Verification items for the finished model (mm, model axes). Give positions to 0.01 mm unless a question says otherwise; leave off trailing zeros. Loops run counter-clockwise (first coordinate to the right, second up) from the corner with the lowest first, then second, coordinate; pieces in that order, holes last. Notation, with made-up numbers: M 50.25,75.5 L 59.25,75.5 A10 ccw 59.25,81.5 Z; hole C 16.25,0.5 d11. An arc over 180 degrees is marked long. Answer in a Markdown table with one row per item.
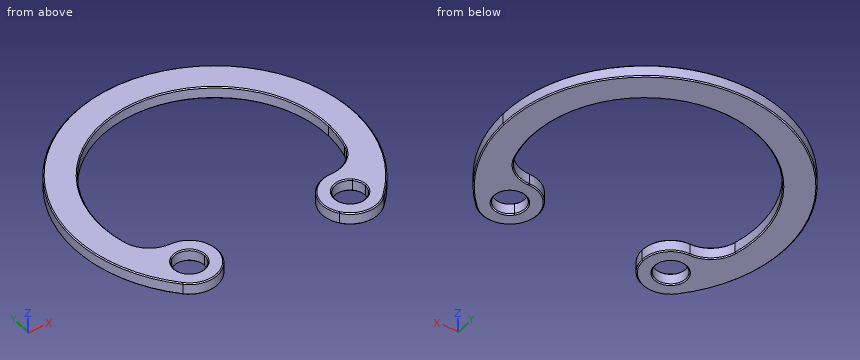
```python
from build123d import *

# Parameters (mm, degrees)
F1_DEPTH = 1.2
F2_R     = 3
F3_SIZE  = 0.1


with BuildPart() as f1:
    # F0 (on Top) → F1 (new body)
    with BuildSketch(Plane.XY):
        with BuildLine():
            ThreePointArc((9.8641395976, -9.8641395976), (12.8881194785, -5.3384338815), (13.95, 0))
            ThreePointArc((13.95, 0), (-5.3384338815, 12.8881194785), (-9.8641395976, -9.8641395976))
            ThreePointArc((-9.8641395976, -9.8641395976), (-10.6786952908, -7.7081070294), (-9.5998734147, -5.6714134412))
            ThreePointArc((-9.5998734147, -5.6714134412), (-2.939720346, 10.7554890306), (11.15, 0))
            ThreePointArc((11.15, 0), (10.7554890306, -2.939720346), (9.5998734147, -5.6714134412))
            ThreePointArc((9.5998734147, -5.6714134412), (10.3985766909, -6.6521228911), (10.6842406102, -7.8842406102))
            ThreePointArc((10.6842406102, -7.8842406102), (10.4711033013, -8.9557542209), (9.8641395976, -9.8641395976))
        make_face()
        with BuildLine():
            ThreePointArc((-5.0842406102, -7.8842406102), (-6.6521228911, -5.3699045296), (-9.5998734147, -5.6714134412))
            ThreePointArc((-9.5998734147, -5.6714134412), (-9.251381225, -6.2237003004), (-8.8711537165, -6.7546377948))
            ThreePointArc((-8.8711537165, -6.7546377948), (-7.2639058858, -6.5185229126), (-6.3842406102, -7.8842406102))
            ThreePointArc((-6.3842406102, -7.8842406102), (-6.4798894748, -8.4113059652), (-6.7546377948, -8.8711537165))
            ThreePointArc((-6.7546377948, -8.8711537165), (-6.2237003004, -9.251381225), (-5.6714134412, -9.5998734147))
            ThreePointArc((-5.6714134412, -9.5998734147), (-5.2350977231, -8.7909059086), (-5.0842406102, -7.8842406102))
        make_face()
        with BuildLine():
            ThreePointArc((-9.5998734147, -5.6714134412), (-10.6786952908, -7.7081070294), (-9.8641395976, -9.8641395976))
            ThreePointArc((-9.8641395976, -9.8641395976), (-7.7081070294, -10.6786952908), (-5.6714134412, -9.5998734147))
            ThreePointArc((-5.6714134412, -9.5998734147), (-6.2237003004, -9.251381225), (-6.7546377948, -8.8711537165))
            ThreePointArc((-6.7546377948, -8.8711537165), (-8.944900782, -8.944900782), (-8.8711537165, -6.7546377948))
            ThreePointArc((-8.8711537165, -6.7546377948), (-9.251381225, -6.2237003004), (-9.5998734147, -5.6714134412))
        make_face()
        with BuildLine():
            ThreePointArc((9.5998734147, -5.6714134412), (5.9043416229, -5.9043416229), (5.6714134412, -9.5998734147))
            ThreePointArc((5.6714134412, -9.5998734147), (6.2237003004, -9.251381225), (6.7546377948, -8.8711537165))
            ThreePointArc((6.7546377948, -8.8711537165), (6.8235804385, -6.8235804385), (8.8711537165, -6.7546377948))
            ThreePointArc((8.8711537165, -6.7546377948), (9.251381225, -6.2237003004), (9.5998734147, -5.6714134412))
        make_face()
        with BuildLine():
            ThreePointArc((5.6714134412, -9.5998734147), (7.7081070294, -10.6786952908), (9.8641395976, -9.8641395976))
            ThreePointArc((9.8641395976, -9.8641395976), (10.4711033013, -8.9557542209), (10.6842406102, -7.8842406102))
            ThreePointArc((10.6842406102, -7.8842406102), (10.3985766909, -6.6521228911), (9.5998734147, -5.6714134412))
            ThreePointArc((9.5998734147, -5.6714134412), (9.251381225, -6.2237003004), (8.8711537165, -6.7546377948))
            ThreePointArc((8.8711537165, -6.7546377948), (9.2499583079, -7.2639058858), (9.3842406102, -7.8842406102))
            ThreePointArc((9.3842406102, -7.8842406102), (8.4113059652, -9.2885917457), (6.7546377948, -8.8711537165))
            ThreePointArc((6.7546377948, -8.8711537165), (6.2237003004, -9.251381225), (5.6714134412, -9.5998734147))
        make_face()
    extrude(amount=F1_DEPTH)

    # F2
    f2_edges = [f1.edges().sort_by_distance(p)[0] for p in [
        (-9.599873, -5.671413, 0.6),
        (9.599873, -5.671413, 0.6),
    ]]
    fillet(f2_edges, radius=F2_R)

    # F3
    f3_edges = [f1.edges().sort_by_distance(p)[0] for p in [
        (-5.297863, -8.956926, 1.2),
        (-9.710143, -4.460557, 1.2),
        (0, 13.95, 1.2),
        (0, 11.15, 1.2),
        (5.297863, -8.956926, 1.2),
        (9.710143, -4.460557, 1.2),
        (-6.897328, -9.013843, 1.2),
        (9.013843, -6.897328, 1.2),
        (0, 11.15, 0),
        (-6.897328, -9.013843, 0),
        (9.013843, -6.897328, 0),
    ]]
    chamfer(f3_edges, length=F3_SIZE)


solid = f1.part
```
Item 1: Scan lines: L1, parallel to Y at x = -8, z = 0.65; L2, parallel to Y at x = 0, z = 0.95; L3, parallel to Y at x = 7, z = 0.95. Record each from-to range of solid material in increasing order. Write a range as [from, to].
Reported:
| item | result |
|---|---|
| L1 | y = [-10.68, -9.38], [-6.39, -5.08], [7.77, 11.43] |
| L2 | y = [11.15, 13.95] |
| L3 | y = [-10.54, -9.1], [-6.67, -5.23], [8.68, 12.07] |
Item 2: Go/stop test with a flat-tipped pin: pin 1 (6 mm diameter, centred on x = -6.5, y = 11.5, fed in from -Z). Record where the tip stops, or that it passes through.
Reported:
| item | result |
|---|---|
| pin 1 | stops at z = 0 |
Item 3: Sectioned sample at B-B (z = 0.65). State how many separate pieces and enclosed holes the cut face has, and give its area (3 significant figures).
Reported:
| item | result |
|---|---|
| separate pieces | 1 |
| enclosed holes | 2 |
| area | 190 mm^2 |
Item 4: Sectioned sample at A-A (x = 0). Record the cut outline in (y, z), and give its area (3 significant figures).
Reported:
| item | result |
|---|---|
| outline | M 11.15,0.1 L 11.25,0 L 13.85,0 L 13.95,0.1 L 13.95,1.1 L 13.85,1.2 L 11.25,1.2 L 11.15,1.1 Z |
| area | 3.34 mm^2 |
